```python
from build123d import *

# Parameters (mm, degrees)
SKETCH1_W                    = 22.6
SKETCH1_H                    = 14.1
BOSS_EXTRUDE1_DEPTH          = 8
SKETCH2_W                    = 33.1
SKETCH2_H                    = 14.1
BOSS_EXTRUDE2_DEPTH          = 2
F_2_0_2_DIAMETER_HOLE1_D     = 2
F_2_0_2_DIAMETER_HOLE1_DEPTH = 2


with BuildPart() as part:
    # Sketch1 → Boss-Extrude1 (new body)
    with BuildSketch(Plane(origin=(0, 0, 0), x_dir=(1, 0, 0), z_dir=(0, 1, 0))):
        Rectangle(SKETCH1_W, SKETCH1_H)
    extrude(amount=BOSS_EXTRUDE1_DEPTH)

    # Sketch2 → Boss-Extrude2 (add)
    with BuildSketch(Plane.XZ):
        Rectangle(SKETCH2_W, SKETCH2_H)
    extrude(amount=BOSS_EXTRUDE2_DEPTH)

    # Ø2.0 (2) Diameter Hole1
    with Locations(Plane(origin=(0, 0, 0), x_dir=(1, 0, 0), z_dir=(0, 1, 0))):
        with Locations((-14.25, 0), (14.25, 0)):
            Hole(F_2_0_2_DIAMETER_HOLE1_D / 2, depth=F_2_0_2_DIAMETER_HOLE1_DEPTH)


solid = part.part
```
Geometry: final body of the model. Coordinates: model frame, mm. A direction names the side the tool comes from. Give positions to 0.01 mm unless a question says otherwise; leave off trailing zeros. Order: outer loops, then holes, each group sorted by start corner. A loop starts at its lowest first (then second) coordinate and runs counter-clockwise, first axis right, second up. Notation, with made-up numbers: M 89.5,75.5 L 148.5,75.5 A21 cw 148.5,114.5 Z; hole C -17.75,79.25 d2. An arc over 180 degrees is marked long. Answer as CSV lines item,"result". Start each with the question number.
1) First-contact query: P1, Ø1.2, axis at x = -14.25, z = 0, coming from the +Y side. Flat tip, straight axial feed; report the tip coordinate or a pass-through.
2) Cut plane C-C (z = 4.5). Output: boundary loops of the cut face in (x, y), then the cut area to 3 significant figures.
3) Mould query, pull axis X, two halves, no side actions, for faces 1 (the flat face through (13, 0, 0)), 2 (the cylindrical face through (13.296, -1.014, -0.3)), 3 (the flat face through (11.3, 4, 0)). Classes: +X half, -X half, draft (parallel to the pull), parting line (faces both ways), or undercut.
4) Cut plane B-B (x = -14.25). Output: boundary loops of the cut face in (y, z).
5) Set-up query: faces 4 (the flat face through (0, -2, 0)), 5 (the flat face through (-13, 0, 0)). Return all of +Z, -Z, +X, -X, +Y, -Y with unobstructed straight access to the full face (end or side cutting, diameter ignored); none if empty.
6) Cut plane D-D (y = 4.75). Output: boundary loops of the cut face in (x, z).
7) Line query: line 1 (Z direction, x = -14.25, y = -0.95); line 2 (X direction, y = 5.5, z = -3.5); line 3 (Y direction, x = 12.5, z = -0.25). Output: solid intervals per line, ascending. Write a range as from..to.
8) Cut plane A-A (z = 0). Output: boundary loops of the cut face in (x, y), then the cut area to 3 significant figures.
Findings below:
1,P1,"passes through"
2,outline,"M -16.55,-2 L 16.55,-2 L 16.55,0 L 11.3,0 L 11.3,8 L -11.3,8 L -11.3,0 L -16.55,0 Z"
2,area,"247 mm²"
3,face 1,"draft"
3,face 2,"undercut"
3,face 3,"+X half"
4,outline,"M -2,-7.05 L 0,-7.05 L 0,-1 L -2,-1 Z; M -2,1 L 0,1 L 0,7.05 L -2,7.05 Z"
5,face 4,"+Z, -Z, +X, -X, -Y"
5,face 5,"+Z, -Z, -X, +Y"
6,outline,"M -11.3,-7.05 L 11.3,-7.05 L 11.3,7.05 L -11.3,7.05 Z"
7,line 1,"z = -7.05..-1, 1..7.05"
7,line 2,"x = -11.3..11.3"
7,line 3,"y = -2..0"
8,outline,"M -16.55,-2 L -15.25,-2 L -15.25,0 L -16.55,0 Z; M -13.25,-2 L 13.25,-2 L 13.25,0 L 11.3,0 L 11.3,8 L -11.3,8 L -11.3,0 L -13.25,0 Z; M 15.25,-2 L 16.55,-2 L 16.55,0 L 15.25,0 Z"
8,area,"239 mm²"
